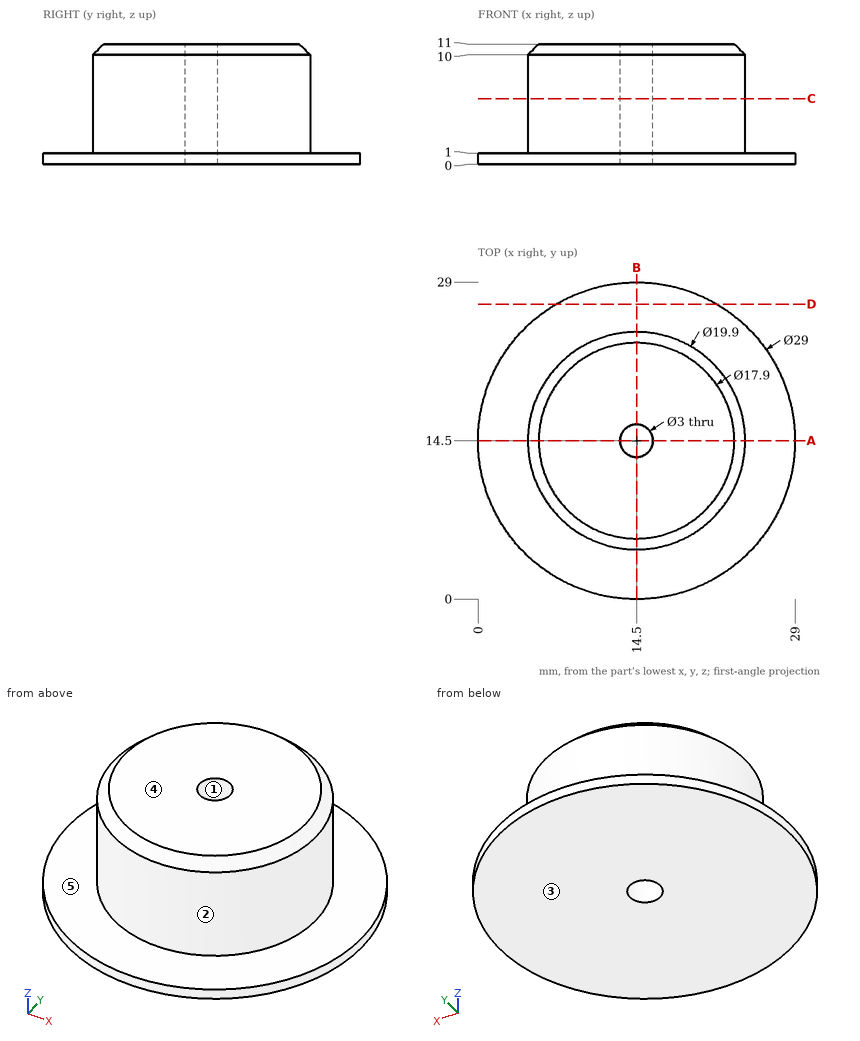
The figure shows three views and two pictorial views of one solid part (mm, origin at its lowest corner). Answer the questions. A direction names the side the tool comes from. Give positions to 0.01 mm unless a question says otherwise; leave off trailing zeros. Order: outer loops, then holes, each group sorted by start corner. A loop starts at its lowest first (then second) coordinate and runs counter-clockwise, first axis right, second up. Notation, with made-up numbers: (25, -6) -> (63, -6) arc R30 ccw to (63, 21) -> close; hole circle Ø7 at (7.5, 17.5). An arc over 180 degrees is marked (long way). Answer as CSV lines item,"result". Start each with the question number.
(1) For a pull along X with two mould halves and no side action, classify the marked faces 1, 2 and 3 as released by +X, released by -X, zero draft, split by the parting line, or undercut.
(2) Section D-D, the plane y = 27 is taken. Write down the section's boundary in (x, z).
(3) Consider line 1 along Y through (x, z) = (14.5, 6.5); line 2 along Z through (x, y) = (20, 5); line 3 along Z through (x, y) = (21.5, 7.75). Determine where each line is inside the solid, lowest interval first.
(4) Which of the six approach directions +Z, -Z, +X, -X, +Y, -Y give full straight-line access (tool end or side, diameter ignored) to the marked faces 4 and 5?
(5) Section C-C, the plane z = 6 is taken. Write down the section's boundary in (x, y), plus the area to 3 significant figures.
(6) Each of these flat-tipped pins is pushed along its axis until it touches: pin 1 Ø1.5 at (y, z) = (12.5, 8.5) entering from +X; pin 2 Ø4 at (y, z) = (17.5, 4) entering from -X; pin 3 Ø6 at (y, z) = (3, 6.5) entering from +X. Where does it stop, or does it pass through?
(7) Section A-A, the plane y = 14.5 is taken. Write down the section's boundary in (x, z).
Entries:
1,face 1,"undercut"
1,face 2,"split by the parting line"
1,face 3,"zero draft"
2,outline,"(7.15, 0) -> (21.85, 0) -> (21.85, 1) -> (7.15, 1) -> close"
3,line 1,"4.55 to 13, 16 to 24.45"
3,line 2,"0 to 1"
3,line 3,"0 to 10.23"
4,face 4,"+Z, +X, -X, +Y, -Y"
4,face 5,"+Z"
5,outline,"circle Ø19.9 at (14.5, 14.5); hole circle Ø3 at (14.5, 14.5)"
5,area,"304 mm²"
6,pin 1,"x = 24.37"
6,pin 2,"x = 4.6"
6,pin 3,"x = 19.67"
7,outline,"(0, 0) -> (13, 0) -> (13, 11) -> (5.55, 11) -> (4.55, 10) -> (4.55, 1) -> (0, 1) -> close; (16, 0) -> (29, 0) -> (29, 1) -> (24.45, 1) -> (24.45, 10) -> (23.45, 11) -> (16, 11) -> close"
